Work out the finished part from the listing and answer in its coordinate system (mm). A direction names the side the tool comes from. Give positions to 0.01 mm unless a question says otherwise; leave off trailing zeros. Loops run counter-clockwise (first coordinate to the right, second up) from the corner with the lowest first, then second, coordinate; pieces in that order, holes last. Notation, with made-up numbers: M 54,-4 L 89,-4 A17 cw 89,2 Z; hole C 84,-6.5 d6. An arc over 180 degrees is marked long. Answer in a Markdown table with one row per item. Add a question column.
from build123d import *

# Parameters (mm, degrees)
ESQUISSE1_W             = 20
ESQUISSE1_H             = 40
BOSS_EXTRU_1_DEPTH      = 15
ESQUISSE2_R             = 1.5
ENL_V_MAT_EXTRU_1_DEPTH = 10
ESQUISSE3_R             = 1.5
ENL_V_MAT_EXTRU_2_DEPTH = 48.16990566
ESQUISSE4_R             = 5
ENL_V_MAT_EXTRU_3_DEPTH = 48.16990566


with BuildPart() as part:
    # Esquisse1 → Boss.-Extru.1 (new body)
    with BuildSketch(Plane.XY):
        with Locations((10, 20)):
            Rectangle(ESQUISSE1_W, ESQUISSE1_H)
    extrude(amount=BOSS_EXTRU_1_DEPTH)

    # Esquisse2 → Enlèv. mat.-Extru.1 (cut)
    with BuildSketch(Plane(origin=(20, 0, 0), x_dir=(0, 0, -1), z_dir=(1, 0, 0))):
        with Locations(Location((-7.5, 35, 0), (0, 0, 90))):
            Circle(ESQUISSE2_R)
        with Locations(Location((-7.5, 7, 0), (0, 0, 90))):
            Circle(ESQUISSE2_R)
    extrude(amount=-ENL_V_MAT_EXTRU_1_DEPTH, mode=Mode.SUBTRACT)

    # Esquisse3 → Enlèv. mat.-Extru.2 (cut, through all)
    with BuildSketch(Plane(origin=(0, 0, 0), x_dir=(-1, 0, 0), z_dir=(0, 0, -1))):
        with Locations((-16, 3)):
            Circle(ESQUISSE3_R)
        with Locations((-3, 3)):
            Circle(ESQUISSE3_R)
    extrude(amount=-ENL_V_MAT_EXTRU_2_DEPTH, mode=Mode.SUBTRACT)

    # Esquisse4 → Enlèv. mat.-Extru.3 (cut, through all)
    with BuildSketch(Plane(origin=(0, 0, 0), x_dir=(-1, 0, 0), z_dir=(0, 0, -1))):
        with Locations((-10, 28)):
            Circle(ESQUISSE4_R)
    extrude(amount=-ENL_V_MAT_EXTRU_3_DEPTH, mode=Mode.SUBTRACT)


solid = part.part
(1) Section A-A, the plane y = 28 is taken. Determine the outline of the cut face in (x, z).
(2) This flat-tipped pin is pushed along its axis until it touches: P1, Ø1.8, axis at y = 35, z = 7.5, coming from the +X side. Where does it stop, or does it pass through?
(3) Consider line 1 along Z through (x, y) = (13.5, 7); line 2 along Y through (x, z) = (3, 5.25); line 3 along Z through (x, y) = (12.5, 7.5). Determine where each line is inside the solid, lowest interval first. Write a range as from..to.
(4) The mould has two halves that part along X. Classify faces 3 (the face through (17.5, 3.07, 7.4)), 4 (the face through (10, 7, 8)), 5 (the face through (10, 40, 7)): pulls with the +X half, pulls with the -X half, needs draft (parallel to the pull), parting line crosses it, or undercut.
(5) Section B-B, the plane x = 3 is taken. Determine the outline of the cut face in (y, z).
(6) Which of the six approach directions +Z, -Z, +X, -X, +Y, -Y give full straight-line access (tool end or side, diameter ignored) to faces 1 (the face through (2.31, 1.67, 7.4)), 2 (the face through (10, 35, 8))?
(7) Section C-C, the plane x = 16.5 is taken. Determine the outline of the cut face in (y, z).
(8) Section D-D, the plane y = 3 is taken. Determine the outline of the cut face in (x, z).
Numbers:
| question | item | result |
|---|---|---|
| 1 | outline | M 0,0 L 5,0 L 5,15 L 0,15 Z; M 15,0 L 20,0 L 20,15 L 15,15 Z |
| 2 | P1 | stops at x = 10 |
| 3 | line 1 | z = 0..6, 9..15 |
| 3 | line 2 | y = 0..1.5, 4.5..40 |
| 3 | line 3 | z = 0..6.09, 8.91..15 |
| 4 | face 3 | undercut |
| 4 | face 4 | pulls with the +X half |
| 4 | face 5 | needs draft |
| 5 | outline | M 0,0 L 1.5,0 L 1.5,15 L 0,15 Z; M 4.5,0 L 40,0 L 40,15 L 4.5,15 Z |
| 6 | face 1 | +Z, -Z |
| 6 | face 2 | +X |
| 7 | outline | M 0,0 L 1.59,0 L 1.59,15 L 0,15 Z; M 4.41,0 L 40,0 L 40,15 L 4.41,15 Z; hole C 7,7.5 d3; hole C 35,7.5 d3 |
| 8 | outline | M 0,0 L 1.5,0 L 1.5,15 L 0,15 Z; M 4.5,0 L 14.5,0 L 14.5,15 L 4.5,15 Z; M 17.5,0 L 20,0 L 20,15 L 17.5,15 Z |
